Input: part model. Units: mm. Frame: model coordinates. Round coordinates to 2 decimals unless told otherwise and drop trailing zeros. Order: outer loops, then holes, each group sorted by start corner. A loop starts at its lowest first (then second) coordinate and runs counter-clockwise, first axis right, second up. Notation, with made-up numbers: (82.25, 24.25) -> (128.25, 24.25) arc R11 cw to (128.25, 45.25) -> close; hole circle Ø8 at (68, 85). An arc over 180 degrees is marked (long way). Use a Markdown table: item, result.
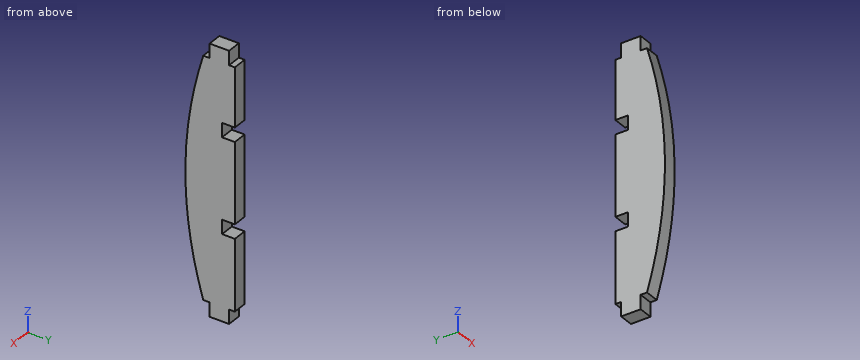
from build123d import *

# Parameters (mm, degrees)
SKICA3_W                 = 50.7
SKICA3_H                 = 6.72
P_IDAT_VYSUNUT_M1_DEPTH  = 3
SKICA3_3_W               = 3
SKICA3_3_H               = 4.15
P_IDAT_VYSUNUT_M2_DEPTH  = 3
SKICA3_4_W               = 3
SKICA3_4_H               = 4.15
P_IDAT_VYSUNUT_M3_DEPTH  = 3
P_IDAT_VYSUNUT_M4_DEPTH  = 3
SKICA5_W                 = 3
SKICA5_H                 = 5.420631859
ODEBRAT_VYSUNUT_M1_DEPTH = 3


with BuildPart() as part:
    # Skica3 → P_idat vysunut_m1 (new body)
    with BuildSketch(Plane(origin=(0, 0, 0), x_dir=(0, 0, -1), z_dir=(1, 0, 0))):
        with Locations((9.501921455, -0.065)):
            Rectangle(SKICA3_W, SKICA3_H)
    extrude(amount=P_IDAT_VYSUNUT_M1_DEPTH)

    # Skica3_3 → P_idat vysunut_m2 (add)
    with BuildSketch(Plane(origin=(0, 0, 0), x_dir=(0, 0, -1), z_dir=(1, 0, 0))):
        with Locations((36.351921455, 0)):
            Rectangle(SKICA3_3_W, SKICA3_3_H)
    extrude(amount=P_IDAT_VYSUNUT_M2_DEPTH)

    # Skica3_4 → P_idat vysunut_m3 (add)
    with BuildSketch(Plane(origin=(0, 0, 0), x_dir=(0, 0, -1), z_dir=(1, 0, 0))):
        with Locations((-17.348078545, 0)):
            Rectangle(SKICA3_4_W, SKICA3_4_H)
    extrude(amount=P_IDAT_VYSUNUT_M3_DEPTH)

    # Skica3_6 → P_idat vysunut_m4 (add)
    with BuildSketch(Plane(origin=(0, 0, 0), x_dir=(0, 0, -1), z_dir=(1, 0, 0))):
        with BuildLine():
            add(Edge.make_bspline(
                [(34.851921455, -3.425), (9.501921455, -11.026061801), (-15.848078545, -3.425)],
                knots=[0, 0, 0, 1, 1, 1], degree=2))
            Line((-15.848078545, -3.425), (34.851921455, -3.425))
        make_face()
    extrude(amount=P_IDAT_VYSUNUT_M4_DEPTH)

    # Skica5 → Odebrat vysunut_m1 (cut)
    with BuildSketch(Plane(origin=(3, 0, 0), x_dir=(0, 0, -1), z_dir=(1, 0, 0))):
        with Locations((-1.848078545, 3.28531593)):
            Rectangle(SKICA5_W, SKICA5_H)
        with Locations((18.241921455, 3.28531593)):
            Rectangle(SKICA5_W, SKICA5_H)
    extrude(amount=-ODEBRAT_VYSUNUT_M1_DEPTH, mode=Mode.SUBTRACT)


solid = part.part
1) Contact query for flat-ended pins moving along their axis: P1, Ø5, axis at y = 1.5, z = -8.5, coming from the -X side; P2, Ø0.6, axis at x = 2, y = 2.5, coming from the -Z side; P3, Ø0.9, axis at x = 1, z = 17.5, coming from the -Y side (3 decimals); P4, Ø1.5, axis at x = 1.5, z = -18.5, coming from the +Y side (3 decimals). Output: stop coordinate, or through.
Answer key:
| item | result |
|---|---|
| P1 | stops at x = 0 |
| P2 | stops at z = -34.85 |
| P3 | stops at y = -2.075 |
| P4 | stops at y = 0.575 |
2) Cut plane A-A on y = 1.5. Return loops of the section in (x, z), and give its area (3 significant figures).
Answer key:
| item | result |
|---|---|
| outline | (0, -37.85) -> (3, -37.85) -> (3, -19.74) -> (0, -19.74) -> close; (0, -16.74) -> (3, -16.74) -> (3, 0.35) -> (0, 0.35) -> close; (0, 3.35) -> (3, 3.35) -> (3, 18.85) -> (0, 18.85) -> close |
| area | 152 mm^2 |
3) Ray query, probe 1 along Z at (x, y) = (0.8, 2.5); probe 2 along Y at (x, z) = (0.75, -9) (3 decimals); probe 3 along Y at (x, z) = (1.4, 13.5) (3 decimals). Return the intervals inside material, ascending.
Answer key:
| item | result |
|---|---|
| probe 1 | z = -34.85 to -19.74, -16.74 to 0.35, 3.35 to 15.85 |
| probe 2 | y = -7.224 to 3.295 |
| probe 3 | y = -4.096 to 3.295 |
